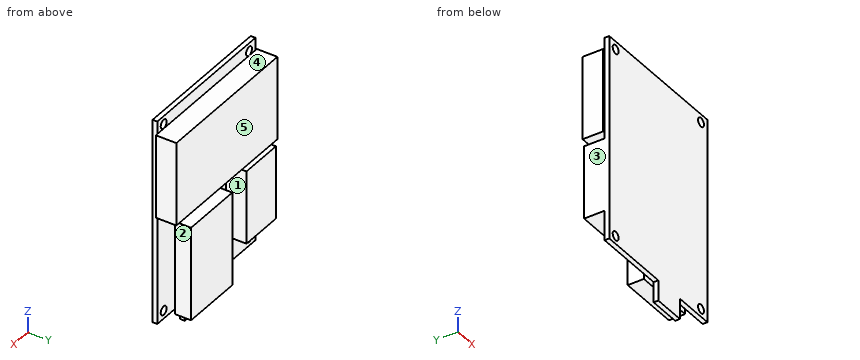
from build123d import *

# Parameters (mm, degrees)
SKETCH_1_W      = 50
SKETCH_1_H      = 70
SKETCH_1_R      = 1.5
EXTRUDE_1_DEPTH = 1.6
SKETCH_3_W      = 51.5
SKETCH_3_H      = 28.5
EXTRUDE_2_DEPTH = 7
SKETCH_4_W      = 15
SKETCH_4_H      = 25
EXTRUDE_3_DEPTH = 7
SKETCH_5_W      = 21
SKETCH_5_H      = 32
EXTRUDE_4_DEPTH = 5.5
SKETCH_6_W      = 11
SKETCH_6_H      = 1.6
EXTRUDE_5_DEPTH = 7


with BuildPart() as part:
    # 草图1 → 凸台-拉伸1 (new body)
    with BuildSketch(Plane(origin=(0, 0, 0), x_dir=(1, 0, 0), z_dir=(0, 1, 0))):
        with Locations((25, 35)):
            Rectangle(SKETCH_1_W, SKETCH_1_H)
        with Locations(Location((3.25, 2.75, 0), (0, 0, 270))):
            Circle(SKETCH_1_R, mode=Mode.SUBTRACT)
        with Locations(Location((46.75, 2.75, 0), (0, 0, 90))):
            Circle(SKETCH_1_R, mode=Mode.SUBTRACT)
        with Locations(Location((46.75, 67.25, 0), (0, 0, 270))):
            Circle(SKETCH_1_R, mode=Mode.SUBTRACT)
        with Locations(Location((3.25, 67.25, 0), (0, 0, 90))):
            Circle(SKETCH_1_R, mode=Mode.SUBTRACT)
    extrude(amount=EXTRUDE_1_DEPTH)

    # 草图3 → 凸台-拉伸2 (add)
    with BuildSketch(Plane(origin=(0, 1.6, 0), x_dir=(1, 0, 0), z_dir=(0, 1, 0))):
        with Locations((25, 18.55)):
            Rectangle(SKETCH_3_W, SKETCH_3_H)
    extrude(amount=EXTRUDE_2_DEPTH)

    # 草图4 → 凸台-拉伸3 (add)
    with BuildSketch(Plane(origin=(0, 1.6, 0), x_dir=(1, 0, 0), z_dir=(0, 1, 0))):
        with Locations((7.5, 47.3)):
            Rectangle(SKETCH_4_W, SKETCH_4_H)
    extrude(amount=EXTRUDE_3_DEPTH)

    # 草图5 → 凸台-拉伸4 (add)
    with BuildSketch(Plane(origin=(0, 1.6, 0), x_dir=(1, 0, 0), z_dir=(0, 1, 0))):
        with Locations((30.5, 55.8)):
            Rectangle(SKETCH_5_W, SKETCH_5_H)
    extrude(amount=EXTRUDE_4_DEPTH)

    # 草图6 → 凸台-拉伸5 (add)
    with BuildSketch(Plane(origin=(0, 0, -70), x_dir=(-1, 0, 0), z_dir=(0, 0, -1))):
        with Locations((-30.5, 0.8)):
            Rectangle(SKETCH_6_W, SKETCH_6_H)
    extrude(amount=EXTRUDE_5_DEPTH)


solid = part.part
Verification items for the finished model (mm, model axes). Face numbers are marked on the shaded views. A direction names the side the tool comes from. Coordinates: 2 decimals unless noted, no trailing zeros. Order: outer loops, then holes, each group sorted by start corner. A loop starts at its lowest first (then second) coordinate and runs counter-clockwise, first axis right, second up. Notation, with made-up numbers: M -10.5,-39.75 L 41.5,-39.75 A16 cw 41.5,-25.75 Z; hole C 57,1.25 d7. An arc over 180 degrees is marked long. One line per item, written item: value. Start each with the question number.
Item 1: Sectioned sample at A-A on z = -67.25. Record the cut outline in (x, y).
Item 2: Thickness scan on probe 1 along X at (y, z) = (1.15, -67.25); probe 2 along Z at (x, y) = (39, 6.25); probe 3 along X at (y, z) = (5.5, -43.5). Record the ranges inside material, lowest first.
Item 3: Sectioned sample at B-B on x = 46.75. Record the cut outline in (y, z).
Item 4: Depth check by flat-ended pin: P1, Ø1.6, axis at x = 35, y = 4.5, coming from the -Z side; P2, Ø4.5, axis at y = 3.5, z = -55.5, coming from the +X side; P3, Ø1.6, axis at y = 4.5, z = -63, coming from the -X side. Enter the tip coordinate at first touch or a pass-through.
Item 5: Access from +Z, -Z, +X, -X, +Y, -Y to the whole of each face (thin tool, end or side, straight path). Record for the marked faces 1, 2, 3, 4 and 5.
Item 6: Sectioned sample at C-C on x = 39.5. Record the cut outline in (y, z).
Item 7: Sectioned sample at D-D on z = -2.75. Record the cut outline in (x, y), then the cut area to 3 significant figures.
Calculated:
1. outline: M 0,0 L 1.75,0 L 1.75,1.6 L 0,1.6 Z; M 4.75,0 L 45.25,0 L 45.25,1.6 L 41,1.6 L 41,7.1 L 20,7.1 L 20,1.6 L 4.75,1.6 Z; M 48.25,0 L 50,0 L 50,1.6 L 48.25,1.6 Z
2. probe 1: 0 to 1.75, 4.75 to 45.25, 48.25 to 50
2. probe 2: -71.8 to -39.8, -32.8 to -4.3
2. probe 3: 0 to 15, 20 to 41
3. outline: M 0,-70 L 1.6,-70 L 1.6,-68.75 L 0,-68.75 Z; M 0,-65.75 L 1.6,-65.75 L 1.6,-32.8 L 8.6,-32.8 L 8.6,-4.3 L 1.6,-4.3 L 1.6,-4.25 L 0,-4.25 Z; M 0,-1.25 L 1.6,-1.25 L 1.6,0 L 0,0 Z
4. P1: z = -71.8
4. P2: x = 50
4. P3: x = 20
5. face 1: -Z, +Y
5. face 2: -Z, +X, +Y
5. face 3: -Z, -X, -Y
5. face 4: +Z, +X, -X, +Y
5. face 5: +Z, -Z, +X, -X, +Y
6. outline: M 0,-70 L 1.6,-70 L 1.6,-71.8 L 7.1,-71.8 L 7.1,-39.8 L 1.6,-39.8 L 1.6,-32.8 L 8.6,-32.8 L 8.6,-4.3 L 1.6,-4.3 L 1.6,0 L 0,0 Z
7. outline: M 0,0 L 1.75,0 L 1.75,1.6 L 0,1.6 Z; M 4.75,0 L 45.25,0 L 45.25,1.6 L 4.75,1.6 Z; M 48.25,0 L 50,0 L 50,1.6 L 48.25,1.6 Z
7. area: 70.4 mm^2
